The listing builds one solid part. Answer for the finished solid, in the listing's coordinates (mm). Face numbers are marked on the shaded views. A direction names the side the tool comes from. Round coordinates to 2 decimals unless told otherwise and drop trailing zeros. Loops run counter-clockwise (first coordinate to the right, second up) from the corner with the lowest first, then second, coordinate; pieces in that order, holes last. Notation, with made-up numbers: (50.5, 3) - (56.5, 3) arc R17 cw to (56.5, 7) - close; hole circle Ø3 at (49.5, -37). An arc over 180 degrees is marked (long way). One line per item, written item: value.
Autodesk Inventor part; units mm, degrees
ref_plane "YZ Plane" through (0, 0, 0) normal (1, 0, 0) x (0, 1, 0)
ref_plane "XZ Plane" through (0, 0, 0) normal (0, 1, 0) x (-1, 0, 0)
ref_plane "XY Plane" through (0, 0, 0) normal (0, 0, 1) x (1, 0, 0)
sketch "sketch" plane through (0, 0, 0) normal (0, 0, 1) x (1, 0, 0)
  line L0 (-21.4, 0) -> (128.4, 0) construction
  line L1 (0, -2) -> (0, 12) construction
  line L2 (0, 10) -> (107, 10)
  line L3 (107, 10) -> (107, 0)
  line L4 (107, 0) -> (0, 0)
  line L5 (0, 0) -> (0, 10)
  line L6 (2, 8.5) -> (11, 8.5)
  line L7 (11, 8.5) -> (11, 1.5)
  line L8 (11, 1.5) -> (2, 1.5)
  line L9 (2, 1.5) -> (2, 8.5)
  circle A0 centre (93.5, 5) radius 1.5
  circle A1 centre (103.5, 5) radius 1.5
  dimension "d0" = 10
  dimension "d1" = 107
  dimension "d2" = 9
  dimension "d3" = 7
  dimension "d4" = 1.5
  dimension "d5" = 2
  dimension "d6" = 3
  dimension "d7" = 3
  dimension "d8" = 3.5
  dimension "d9" = 10
  dimension "d10" = 5
  dimension "d11" = 5
extrude "body" add sketch "sketch" along normal blind 3 contours L2 L3 L4 L5 | L6 L7 L8 L9
extrude "button" add sketch "sketch" against normal blind 8 contours L6 L7 L8 L9
sketch "button_sketch" plane through (0, 0, 3) normal (0, 0, 1) x (1, 0, 0)
  line L0 (11, 1.5) -> (2, 1.5)
  line L1 (11, 8.5) -> (2, 8.5)
  line L2 (2, 8.5) -> (2, 1.5)
  line L3 (11, 1.5) -> (11, 8.5)
  circle A0 centre (6.5, 5) radius 1.5
  line L4 (107, 10) -> (0, 10)
  point P0 (0, 0)
  dimension "d16" = 3
  dimension "d17" = 5
  dimension "d18" = 4.5
extrude "bolt" cut sketch "button_sketch" against normal blind 8 contours A0
fillet "모깎기1" radius 1.5 8 edges at (6.5, 1.5, -8) (2, 5, -8) (11, 5, -8) (6.5, 8.5, -8) (11, 1.5, -4) (2, 1.5, -4) (2, 8.5, -4) (11, 8.5, -4)
equation "\"d4\" = -0.5 * d3 + 0.5 * d0"
equation "\"d17\" = 0.5 * d0"
equation "\"d18\" = 0.5 * d2"
properties part number "button_bar"
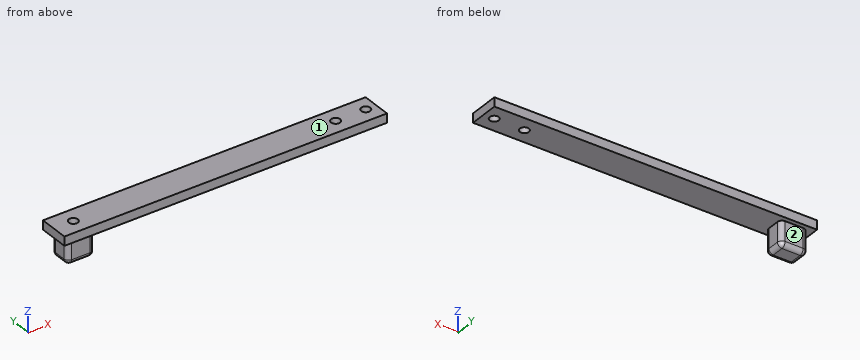
1) For the marked faces 1 and 2, determine the directions among +Z, -Z, +X, -X, +Y, -Y from which every point of the face is accessible in a straight line to the end or side of a thin tool.
Final values:
face 1: +Z, +X, -X, +Y, -Y
face 2: -Z, +X, -X, +Y
2) A cutting plane is placed at D-D on x = 26.5. Give the vertices of the cut face in (y, z), and give its area (3 significant figures).
Final values:
outline: (0, 0) - (10, 0) - (10, 3) - (0, 3) - close
area: 30.0 mm2
3) A cutting plane is placed at B-B on z = -3. Give the vertices of the cut face in (x, y), and give its area (3 significant figures).
Final values:
outline: (2, 3) arc R1.5 ccw to (3.5, 1.5) - (9.5, 1.5) arc R1.5 ccw to (11, 3) - (11, 7) arc R1.5 ccw to (9.5, 8.5) - (3.5, 8.5) arc R1.5 ccw to (2, 7) - close; hole circle Ø3 at (6.5, 5)
area: 54.0 mm2
4) Each of these flat-tipped pins is pushed along its axis until it touches: pin 1 Ø1 at (x, y) = (56, 2.5) entering from -Z; pin 2 Ø5 at (x, z) = (7.5, -5) entering from +Y; pin 3 Ø2.5 at (x, y) = (93.5, 5) entering from +Z; pin 4 Ø3 at (y, z) = (5.5, -2.5) entering from +X. Where does it stop, or does it pass through?
Final values:
pin 1: z = 0
pin 2: y = 8.5
pin 3: through
pin 4: x = 11
5) Consider L1, parallel to Y at x = 6.5, z = 2; L2, parallel to X at y = 5.25, z = 2.5; L3, parallel to Y at x = 6.5, z = -1. Determine where each line is inside the solid, lowest interval first.
Final values:
L1: 0 to 3.5, 6.5 to 10
L2: 0 to 5.02, 7.98 to 92.02, 94.98 to 102.02, 104.98 to 107
L3: 1.5 to 3.5, 6.5 to 8.5
6) A cutting plane is placed at A-A on x = 103.5. Give the vertices of the cut face in (y, z).
Final values:
outline: (0, 0) - (3.5, 0) - (3.5, 3) - (0, 3) - close; (6.5, 0) - (10, 0) - (10, 3) - (6.5, 3) - close
7) A cutting plane is placed at C-C on x = 6.5. Give the vertices of the cut face in (y, z), and give its area (3 significant figures).
Final values:
outline: (0, 0) - (1.5, 0) - (1.5, -6.5) arc R1.5 ccw to (3, -8) - (7, -8) arc R1.5 ccw to (8.5, -6.5) - (8.5, 0) - (10, 0) - (10, 3) - (6.5, 3) - (6.5, -5) - (3.5, -5) - (3.5, 3) - (0, 3) - close
area: 61.0 mm2
